Geometry: final body of the model. Coordinates: model frame, mm. A direction names the side the tool comes from. Give positions to 0.01 mm unless a question says otherwise; leave off trailing zeros. Loops run counter-clockwise (first coordinate to the right, second up) from the corner with the lowest first, then second, coordinate; pieces in that order, holes last.
1. Material intervals for line 1 along Z through (x, y) = (0.75, -2); line 2 along X through (y, z) = (8, -0.25); line 3 along Y through (x, z) = (0.75, -3.25), sorted ascending.
2. Section B-B, the plane z = 0. Output: boundary loops of the cut face in (x, y).
3. Draft query along Z for faces 1 (the face through (2, 22.5, 4)), 2 (the face through (0, -3, 1.5)), 3 (the face through (-1.08, 2.96, 4.88)). Return one class per face: +Z half, -Z half, draft (parallel to the pull), parting line (faces both ways), or undercut.
4. Section D-D, the plane y = 4. Output: boundary loops of the cut face in (x, z).
5. Section C-C, the plane y = 8. Output: boundary loops of the cut face in (x, z), then the cut area to 3 significant figures.
6. Section A-A, the plane x = 0. Output: boundary loops of the cut face in (y, z).
7. Access query for faces 4 (the face through (-0.867, 24.472, 3.905)), 5 (the face through (0, -3, -2)), 6 (the face through (1.6, 6, 4.9)), 7 (the face through (0, -3, 2)), 8 (the face through (0, -3, -1.5)). Directions: +Z, -Z, +X, -X, +Y, -Y. A direction counts if a zero-diameter tool reaches every point of the face in a straight line with its end or side. Return the directions, or none.
8. First-contact query: P1, Ø2, axis at x = 0, y = -4.5, coming from the -Z side; P2, Ø4, axis at y = 2.5, z = 3, coming from the -X side; P3, Ø0.6, axis at y = -2, z = -2, coming from the +X side. Flat tips, straight axial feed; report the tip coordinate or a pass-through.
from build123d import *

# Parameters (mm, degrees)
ESBO_O2_W                = 2
ESBO_O2_H                = 0.5
RESSALTO_EXTRUS_O1_DEPTH = 6


with BuildPart() as part:
    # Esboço1 → Revolução1 (revolve)
    with BuildSketch(Plane.XY):
        Polygon((0, 26.5), (4, 26.5), (4, 22.5), (4.891304348, 22.5), (7, 22), (7, 12), (5.5, 12), (5.5, 6), (5, 6), (5, 0), (0, 0), align=None)
    revolve(axis=Axis((0, 0, 0), (0, 1, 0)))

    # Esboço2 → Ressalto-extrusão1 (add)
    with BuildSketch(Plane.XZ):
        with Locations((0, -1.75)):
            Rectangle(ESBO_O2_W, ESBO_O2_H)
        with Locations((0, 1.75)):
            Rectangle(ESBO_O2_W, ESBO_O2_H)
    extrude(amount=RESSALTO_EXTRUS_O1_DEPTH)


solid = part.part
Answers below:
1. line 1: z = -2 to -1.5, 1.5 to 2
1. line 2: x = -5.49 to 5.49
1. line 3: y = 0 to 26.5
2. outline: (-7, 12) - (-5.5, 12) - (-5.5, 6) - (-5, 6) - (-5, 0) - (5, 0) - (5, 6) - (5.5, 6) - (5.5, 12) - (7, 12) - (7, 22) - (4.89, 22.5) - (4, 22.5) - (4, 26.5) - (-4, 26.5) - (-4, 22.5) - (-4.89, 22.5) - (-7, 22) - close
3. face 1: draft
3. face 2: undercut
3. face 3: parting line
4. outline: circle Ø10 at (0, 0)
5. outline: circle Ø11 at (0, 0)
5. area: 95.0 mm2
6. outline: (-6, -2) - (0, -2) - (0, -5) - (6, -5) - (6, -5.5) - (12, -5.5) - (12, -7) - (22, -7) - (22.5, -4.89) - (22.5, -4) - (26.5, -4) - (26.5, 4) - (22.5, 4) - (22.5, 4.89) - (22, 7) - (12, 7) - (12, 5.5) - (6, 5.5) - (6, 5) - (0, 5) - (0, 2) - (-6, 2) - (-6, 1.5) - (0, 1.5) - (0, -1.5) - (-6, -1.5) - close
7. face 4: +Y
7. face 5: -Z, +X, -X, -Y
7. face 6: -Y
7. face 7: +Z, +X, -X, -Y
7. face 8: +X, -X, -Y
8. P1: stops at z = -2
8. P2: stops at x = -4.9
8. P3: stops at x = 1
